```python
from build123d import *

# Parameters (mm, degrees)
BOSS_EXTRUDE1_DEPTH = 32.5
FILLET1_R           = 5
BOSS_EXTRUDE2_DEPTH = 3
FILLET2_R           = 1.5
FILLET3_R           = 1.5
CUT_EXTRUDE1_REACH  = 51.168


# Some blends are built 0.0001 mm under size
with BuildPart() as part:
    # Sketch1 → Boss-Extrude1 (new body)
    with BuildSketch(Plane.XY):
        Polygon((7.518400000000005, 16.559701585568554), (7.518400000000011, -33.66819896343934), (3.199999999999987, -36.16142836590783), (3.1999999999999793, 19.05293098803705), align=None)
    extrude(amount=-BOSS_EXTRUDE1_DEPTH)

    # Fillet1
    # the kernel refuses this fillet: 5 mm, written as the material it takes off along each edge
    with BuildSketch(Plane(origin=(7.518400000000003, 28.94301228989969, 0), x_dir=(0, 0, -1), z_dir=(1.2e-16, -1, 0))) as fillet1_piece_1:
        with BuildLine():
            CenterArc((4.953324281732454, -5), FILLET1_R, 90, 82.16504398350045)
            Line((2.931e-14, -4.318400000000029), (-0.09906648563461919, -4.3047680000000295))
            ThreePointArc((-0.09906648563461919, -4.3047680000000295), (-0.1, -2.1592000000000144), (-0.1, 0))
            Line((-0.1, 0), (0, 0.09999999999999964))
            Line((0, 0.09999999999999964), (4.953324281732454, 0.09999999999999964))
            Line((4.953324281732454, 0.09999999999999964), (4.953324281732454, 0))
        make_face()
    extrude(amount=74.99452195767016, mode=Mode.SUBTRACT)

    # Sketch3 → Boss-Extrude2 (add)
    with BuildSketch(Plane(origin=(7.518400000000007, 9.1e-16, 0), x_dir=(0, 0, -1), z_dir=(1, 1.2e-16, 0))):
        Polygon((8.953324281732419, -1.5542486889353926), (11.953324281732419, -1.554248688935389), (11.95332428173242, -15.55424868893539), (8.95332428173242, -15.55424868893539), align=None)
    extrude(amount=BOSS_EXTRUDE2_DEPTH)

    # Fillet2
    fillet2_edges = [part.edges().sort_by_distance(p)[0] for p in [
        (10.518400000000009, -8.55424868893539, -8.95332428173242),
        (10.518400000000009, -15.554248688935388, -10.45332428173242),
        (10.518400000000009, -8.554248688935386, -11.95332428173242),
        (10.518400000000007, -1.5542486889353895, -10.453324281732419),
    ]]
    fillet(fillet2_edges, radius=FILLET2_R - 0.0001)  # a hair under: the kernel refuses the full size

    # Fillet3
    # the kernel refuses this fillet: 1.5 mm, written as the material it takes off along each edge
    with BuildSketch(Plane(origin=(10.518400000000009, -14.05424868893539, -10.45332428173242), x_dir=(1.2e-16, -1, 0), z_dir=(0, 0, 1))) as fillet3_piece_1:
        with BuildLine():
            CenterArc((9.999999999999e-05, -1.4999), 1.4999, 0, 90)
            Line((1.5, -1.4999), (1.5, 0))
            Line((1.5, 0), (9.999999999999e-05, 0))
        make_face()
    revolve(axis=Axis((10.518400000000009, -14.05424868893539, -10.45332428173242), (1, 1.2e-16, 0)), revolution_arc=90.00000000000001, mode=Mode.SUBTRACT)
    with BuildSketch(Plane(origin=(10.518400000000009, -14.054248688935388, -10.45332428173242), x_dir=(0, -1.3e-16, 1), z_dir=(-1.2e-16, 1, 1.3e-16))) as fillet3_piece_2:
        with BuildLine():
            CenterArc((9.999999999999e-05, -1.4999), 1.4999, 0, 90)
            Line((1.5, -1.4999), (1.5, 0))
            Line((1.5, 0), (9.999999999999e-05, 0))
        make_face()
    revolve(axis=Axis((10.518400000000009, -14.054248688935388, -10.45332428173242), (1, 1.2e-16, 0)), revolution_arc=90, mode=Mode.SUBTRACT)
    with BuildSketch(Plane(origin=(10.518400000000009, -3.05424868893539, -10.453324281732419), x_dir=(0, 1.3e-16, -1), z_dir=(1.2e-16, -1, -1.3e-16))) as fillet3_piece_3:
        with BuildLine():
            CenterArc((9.999999999999e-05, -1.4999), 1.4999, 0, 90)
            Line((1.5, -1.4999), (1.5, 0))
            Line((1.5, 0), (9.999999999999e-05, 0))
        make_face()
    revolve(axis=Axis((10.518400000000009, -3.05424868893539, -10.453324281732419), (1, 1.2e-16, 0)), revolution_arc=90.00000000000006, mode=Mode.SUBTRACT)
    with BuildSketch(Plane(origin=(10.518400000000009, -3.05424868893539, -10.453324281732419), x_dir=(-1.2e-16, 1, 1.18e-15), z_dir=(0, 1.18e-15, -1))) as fillet3_piece_4:
        with BuildLine():
            CenterArc((9.999999999999e-05, -1.4999), 1.4999, 0, 90)
            Line((1.5, -1.4999), (1.5, 0))
            Line((1.5, 0), (9.999999999999e-05, 0))
        make_face()
    revolve(axis=Axis((10.518400000000009, -3.05424868893539, -10.453324281732419), (1, 1.2e-16, 0)), revolution_arc=89.99999999999994, mode=Mode.SUBTRACT)
    with BuildSketch(Plane(origin=(7.518400000000007, -1.5542486889353917, -8.953324281732419), x_dir=(0, 1.18e-15, -1), z_dir=(1, 1.2e-16, 0))) as fillet3_piece_5:
        with BuildLine():
            CenterArc((FILLET3_R, -FILLET3_R), FILLET3_R, 90, 89.99999999999986)
            Line((-1.78e-15, -FILLET3_R), (-FILLET3_R * 0.02, -FILLET3_R))
            Line((-FILLET3_R * 0.02, -FILLET3_R), (-FILLET3_R * 0.02, FILLET3_R * 0.02))
            Line((-FILLET3_R * 0.02, FILLET3_R * 0.02), (FILLET3_R, FILLET3_R * 0.02))
            Line((FILLET3_R, FILLET3_R * 0.02), (FILLET3_R, 0))
        make_face()
    extrude(amount=3, mode=Mode.SUBTRACT)
    with BuildSketch(Plane(origin=(7.518400000000007, -1.5542486889353881, -11.953324281732419), x_dir=(0, -1.18e-15, 1), z_dir=(1, 1.2e-16, 0))) as fillet3_piece_6:
        with BuildLine():
            CenterArc((FILLET3_R, FILLET3_R), FILLET3_R, 179.99999999999994, 90.00000000000006)
            Line((1.78e-15, FILLET3_R), (-FILLET3_R * 0.02, FILLET3_R))
            Line((-FILLET3_R * 0.02, FILLET3_R), (-FILLET3_R * 0.02, -FILLET3_R * 0.02))
            Line((-FILLET3_R * 0.02, -FILLET3_R * 0.02), (FILLET3_R, -FILLET3_R * 0.02))
            Line((FILLET3_R, -FILLET3_R * 0.02), (FILLET3_R, 0))
        make_face()
    extrude(amount=3, mode=Mode.SUBTRACT)
    with BuildSketch(Plane(origin=(7.518400000000009, -15.554248688935388, -11.95332428173242), x_dir=(-1.2e-16, 1, 0), z_dir=(1, 1.2e-16, 0))) as fillet3_piece_7:
        with BuildLine():
            CenterArc((FILLET3_R, FILLET3_R), FILLET3_R, 180, 90)
            Line((-1.78e-15, FILLET3_R), (-FILLET3_R * 0.02, FILLET3_R))
            Line((-FILLET3_R * 0.02, FILLET3_R), (-FILLET3_R * 0.02, -FILLET3_R * 0.02))
            Line((-FILLET3_R * 0.02, -FILLET3_R * 0.02), (FILLET3_R, -FILLET3_R * 0.02))
            Line((FILLET3_R, -FILLET3_R * 0.02), (FILLET3_R, 0))
        make_face()
    extrude(amount=3, mode=Mode.SUBTRACT)
    with BuildSketch(Plane(origin=(7.518400000000009, -15.554248688935388, -8.95332428173242), x_dir=(-1.2e-16, 1, 0), z_dir=(1, 1.2e-16, 0))) as fillet3_piece_8:
        with BuildLine():
            CenterArc((FILLET3_R, -FILLET3_R), FILLET3_R, 90, 90)
            Line((0, -FILLET3_R), (-FILLET3_R * 0.02, -FILLET3_R))
            Line((-FILLET3_R * 0.02, -FILLET3_R), (-FILLET3_R * 0.02, FILLET3_R * 0.02))
            Line((-FILLET3_R * 0.02, FILLET3_R * 0.02), (FILLET3_R, FILLET3_R * 0.02))
            Line((FILLET3_R, FILLET3_R * 0.02), (FILLET3_R, 0))
        make_face()
    extrude(amount=3, mode=Mode.SUBTRACT)
    fillet3_2_edges = [part.edges().sort_by_distance(p)[0] for p in [
        (7.518400000000008, -8.554248688935388, -8.953324281732419),
        (7.518400000000008, -8.55424868893539, -11.95332428173242),
    ]]
    fillet(fillet3_2_edges, radius=FILLET3_R)

    # Sketch4 → Cut-Extrude1 (cut, up to next)
    with BuildSketch(Plane.ZY.offset(-3.199999999999982), mode=Mode.PRIVATE) as cut_extrude1_sk1:
        with BuildLine():
            Line((-0.28410604604419637, -36.161428365907824), (0, -36.16142836590783))
            Line((0, -36.16142836590783), (6.94e-15, -34.499999999999986))
            ThreePointArc((6.94e-15, -34.499999999999986), (-0.07153828412053453, -35.34277227951001), (-0.28410604604419637, -36.161428365907824))
        make_face()
    cut_extrude1_tool1 = extrude(cut_extrude1_sk1.sketch, amount=-CUT_EXTRUDE1_REACH, mode=Mode.PRIVATE) & part.part
    add(cut_extrude1_tool1.solids().sort_by_distance((3.2, -35.748468, -0.0848))[0], mode=Mode.SUBTRACT)


solid = part.part
```
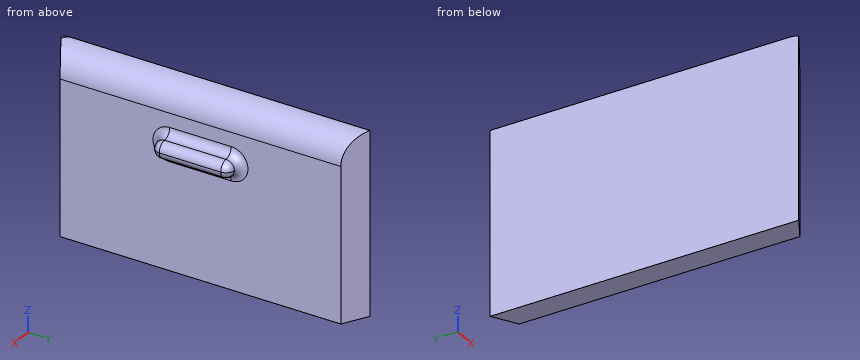
Verification items for the finished model (mm, model axes). Give positions to 0.01 mm unless a question says otherwise; leave off trailing zeros. Write each loop counter-clockwise with the first axis right and the second up, starting at its lowest first coordinate (ties: lowest second). Pieces come first, ordered by that corner, then holes. Notation, with made-up numbers: M 82,-3 L 107,-3 A8 ccw 107,11 Z; hole C -38,21.25 d8. An arc over 180 degrees is marked long. One line per question, with ' | ' between items.
1) Gauge pin test, flat end, axial feed: pin 1 Ø2 at (y, z) = (-11.5, -22) entering from +X. Record the tip position at first contact, or that the pin passes through.
Result:
pin 1: stops at x = 7.52
2) Thickness scan on line 1 along X through (y, z) = (-25, -7.5); line 2 along Z through (x, y) = (3.5, -8); line 3 along X through (y, z) = (17.5, -4). Record the ranges inside material, lowest first. Write a range as [from, to].
Result:
line 1: x = [3.2, 7.52] | line 2: z = [-32.5, -0.05] | line 3: x = [3.2, 5.89]
3) Section check C-C on x = 4.75. Enter the section's corners in (y, z).
Result:
outline: M -35.27,-32.5 L 18.16,-32.5 L 18.16,-0.48 L -35.27,-0.48 Z
4) Section check B-B on z = -18. Enter the section's corners in (x, y), plus the area to 3 significant figures.
Result:
outline: M 3.2,-36.16 L 7.52,-33.67 L 7.52,16.56 L 3.2,19.05 Z | area: 228 mm2
